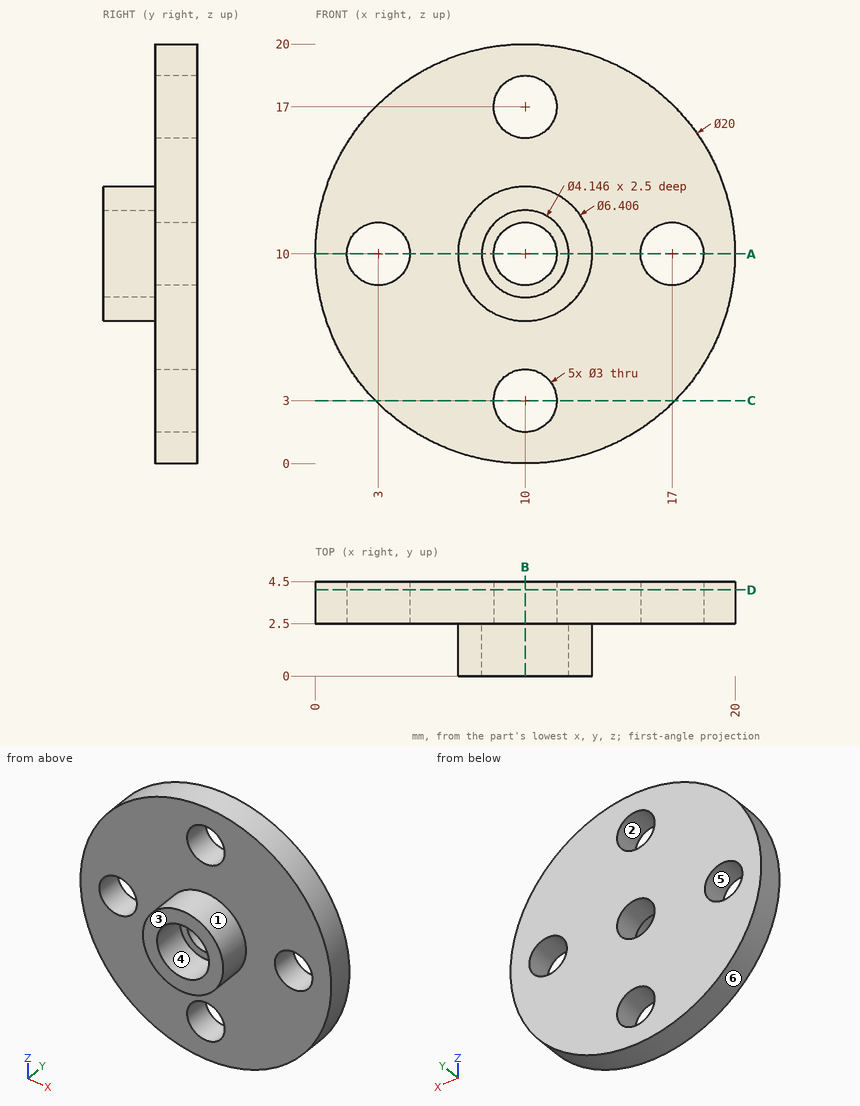
The drawing under review shows one solid part. Ordinate dimensions are in mm from its lowest x, y, z. A direction names the side the tool comes from. Round coordinates to 2 decimals unless told otherwise and drop trailing zeros. Loops run counter-clockwise (first coordinate to the right, second up) from the corner with the lowest first, then second, coordinate; pieces in that order, holes last. Notation, with made-up numbers: (9.5, -2.75) - (36.5, -2.75) arc R33 ccw to (36.5, 27.25) - close; hole circle Ø10 at (-6.75, 20). An arc over 180 degrees is marked (long way). Use a Markdown table: item, result. Add a question column.
Q1. Machinability: for the marked faces 1 and 2, which of the approach directions +Z, -Z, +X, -X, +Y, -Y give a long, thin tool a straight path to every point of the face, cutting with its end or side? Answer none if there is none.
Q2. Add section B-B (x = 10). State the section outline as (y, z) points.
Q3. Add section A-A (z = 10). State the section outline as (x, y) points.
Q4. The part is to be moulded in two halves that separate along Z. For the marked faces 3, 4, 5 and 6, say which applies: pulls with the +Z half, pulls with the -Z half, needs draft (parallel to the pull), parting line crosses it, or undercut.
Q5. Insertion check: pin 1 Ø3.5 at (x, z) = (10, 3) entering from -Y; pin 2 Ø1.5 at (y, z) = (2.5, 7.5) entering from -X. Each pin has a flat end and moves straight along its axis. Give the tip position at first contact, or say it passes through.
Q6. Add section D-D (y = 4.1). State the section outline as (x, z) points, plus the area to 3 significant figures.
Q7. Add section C-C (z = 3). State the section outline as (x, y) points.
Q8. For probe 1 along X at (y, z) = (3.7, 10); probe 2 along Y at (x, z) = (15.25, 10.75); probe 3 along Z at (x, y) = (10.5, 0.8) (1 decimal), list the stretches that pass through material, from the lowest coordinate up.
Worked answers:
| question | item | result |
|---|---|---|
| 1 | face 1 | -Y |
| 1 | face 2 | +Y, -Y |
| 2 | outline | (0, 6.8) - (2.5, 6.8) - (2.5, 4.5) - (4.5, 4.5) - (4.5, 8.5) - (2.5, 8.5) - (2.5, 7.93) - (0, 7.93) - close; (0, 12.07) - (2.5, 12.07) - (2.5, 11.5) - (4.5, 11.5) - (4.5, 15.5) - (2.5, 15.5) - (2.5, 13.2) - (0, 13.2) - close; (2.5, 0) - (4.5, 0) - (4.5, 1.5) - (2.5, 1.5) - close; (2.5, 18.5) - (4.5, 18.5) - (4.5, 20) - (2.5, 20) - close |
| 3 | outline | (0, 2.5) - (1.5, 2.5) - (1.5, 4.5) - (0, 4.5) - close; (4.5, 2.5) - (6.8, 2.5) - (6.8, 0) - (7.93, 0) - (7.93, 2.5) - (8.5, 2.5) - (8.5, 4.5) - (4.5, 4.5) - close; (11.5, 2.5) - (12.07, 2.5) - (12.07, 0) - (13.2, 0) - (13.2, 2.5) - (15.5, 2.5) - (15.5, 4.5) - (11.5, 4.5) - close; (18.5, 2.5) - (20, 2.5) - (20, 4.5) - (18.5, 4.5) - close |
| 4 | face 3 | needs draft |
| 4 | face 4 | undercut |
| 4 | face 5 | undercut |
| 4 | face 6 | parting line crosses it |
| 5 | pin 1 | y = 2.5 |
| 5 | pin 2 | x = 0.15 |
| 6 | outline | circle Ø20 at (10, 10); hole circle Ø3 at (3, 10); hole circle Ø3 at (10, 3); hole circle Ø3 at (10, 10); hole circle Ø3 at (10, 17); hole circle Ø3 at (17, 10) |
| 6 | area | 279 mm² |
| 7 | outline | (2.86, 2.5) - (8.5, 2.5) - (8.5, 4.5) - (2.86, 4.5) - close; (11.5, 2.5) - (17.14, 2.5) - (17.14, 4.5) - (11.5, 4.5) - close |
| 8 | probe 1 | 0 to 1.5, 4.5 to 8.5, 11.5 to 15.5, 18.5 to 20 |
| 8 | probe 2 | 2.5 to 4.5 |
| 8 | probe 3 | 6.8 to 8, 12 to 13.2 |
